The model under review builds one solid part; all positions refer to its coordinate system, in mm. A direction names the side the tool comes from. Coordinates: 2 decimals unless noted, no trailing zeros. Loops run counter-clockwise (first coordinate to the right, second up) from the corner with the lowest first, then second, coordinate; pieces in that order, holes last. Notation, with made-up numbers: M 23,79 L 76,79 A25 ccw 76,111 Z; hole C 52,70 d10. An arc over 180 degrees is marked long. Return JSON: item names as keys, results as strings.
```python
from build123d import *

# Parameters (mm, degrees)
F1_DEPTH       = 25.4
F2_T           = -2.54
F4_D           = 6.35
F4_DEPTH       = 12.7
F4_CSINK_D     = 12.7
F4_CSINK_ANGLE = 90


with BuildPart() as f1:
    # F0 (on Top) → F1 (new body)
    with BuildSketch(Plane.XY):
        with BuildLine():
            ThreePointArc((-57.059065, -53.702373), (-55.199193, -58.192501), (-50.709065, -60.052373))
            Line((-50.709065, -60.052373), (17.889393, -60.052373))
            Line((17.889393, -60.052373), (17.889393, 27.981024))
            Line((17.889393, 27.981024), (-57.059065, 27.981024))
            Line((-57.059065, 27.981024), (-57.059065, -53.702373))
        make_face()
    extrude(amount=F1_DEPTH)

    # F2
    f2_openings = [f1.faces().sort_by_distance(p)[0] for p in [
        (-19.537486, -15.979733, 25.4),
    ]]
    offset(amount=F2_T, openings=f2_openings)

    # F4
    with Locations(Plane.YZ.offset(17.889393)):
        with Locations((-46.142266, 14.274741), (-20.742266, 14.274741)):
            CounterSinkHole(F4_D / 2, F4_CSINK_D / 2, depth=F4_DEPTH, counter_sink_angle=F4_CSINK_ANGLE)


solid = f1.part
```
1. Add section A-A on z = 5.5. Give the boundary of the cut face in (x, y).
Check values:
{"outline": "M -57.06,-53.7 A6.35 ccw -50.71,-60.05 L 17.89,-60.05 L 17.89,27.98 L -57.06,27.98 Z; hole M -54.52,-53.7 A3.81 ccw -50.71,-57.51 L 15.35,-57.51 L 15.35,25.44 L -54.52,25.44 Z"}
2. To check wall thickness, follow line 1 (X direction, y = -2.5, z = 19.5); line 2 (Y direction, x = -41, z = 4); line 3 (Z direction, x = -31.5, y = -17). State the ranges of each line that lie inside material, in increasing order.
Check values:
{"line 1": "-57.06 to -54.52, 15.35 to 17.89", "line 2": "-60.05 to -57.51, 25.44 to 27.98", "line 3": "0 to 2.54"}
3. The part is to be moulded in two halves that separate along Z. For faces 1 (the face through (15.5, -45.6, 18.2)), 2 (the face through (15.5, -20.2, 18.2)), 3 (the face through (-19, 27.981, 13)), 4 (the face through (-20, -15, 0)), say which applies: released by +Z, released by -Z, zero draft, split by the parting line, or undercut.
Check values:
{"face 1": "undercut", "face 2": "undercut", "face 3": "zero draft", "face 4": "released by -Z"}
4. Machinability: for faces 5 (the face through (-17, -60.052, 13)), 6 (the face through (15.349, -16.6, 13.8)), which of the approach directions +Z, -Z, +X, -X, +Y, -Y give a long, thin tool a straight path to every point of the face, cutting with its end or side? Answer none if there is none.
Check values:
{"face 5": "+Z, -Z, +X, -X, -Y", "face 6": "+Z"}
5. Add section B-B on x = 1. Give the boundary of the cut face in (y, z), plus the area to 3 significant figures.
Check values:
{"outline": "M -60.05,0 L 27.98,0 L 27.98,25.4 L 25.44,25.4 L 25.44,2.54 L -57.51,2.54 L -57.51,25.4 L -60.05,25.4 Z", "area": "340 mm²"}
6. Insertion check: pin 1 Ø6 at (x, y) = (-42, -11.5) entering from +Z. The pin has a flat end and moves straight along its axis. Give the tip position at first contact, or say it passes through.
Check values:
{"pin 1": "z = 2.54"}
7. Add section C-C on y = -30.5. Give the boundary of the cut face in (x, z).
Check values:
{"outline": "M -57.06,0 L 17.89,0 L 17.89,25.4 L 15.35,25.4 L 15.35,2.54 L -54.52,2.54 L -54.52,25.4 L -57.06,25.4 Z"}
